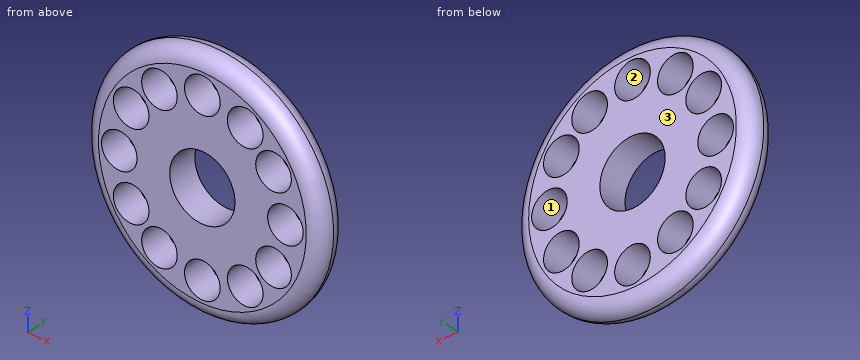
```python
from build123d import *

# Parameters (mm, degrees)
F0_R     = 40
F1_DEPTH = 5
F3_D     = 22
F4_D     = 12
F5_R     = 4.99999


# Not quite as in the source:
# - a fillet or chamfer is up to 0.001 mm smaller than in the source, because OpenCascade refuses the exact size
# - a feature names something its author has since deleted; it is built from what else it names


with BuildPart() as f1:
    # F0 (on Front) → F1 (new body, symmetric)
    with BuildSketch(Plane.XZ):
        Circle(F0_R)
    extrude(amount=F1_DEPTH, both=True)

    # F3 (through all)
    with Locations(Plane.XZ.offset(5)):
        with Locations((0, 0)):
            Hole(F3_D / 2)

    # F4 (through all)
    with Locations(Plane.XZ.offset(5)):
        with Locations((-28, 0), (0, 28), (28, 0), (0, -28), (-23.9821428571, 14.4518796002), (-14.4518796002, 23.9821428571), (14.4518796002, 23.9821428571), (23.9821428571, 14.4518796002), (23.9821428571, -14.4518796002), (-14.4518796002, -23.9821428571), (14.4518796002, -23.9821428571), (-23.9821428571, -14.4518796002)):
            Hole(F4_D / 2)

    # F5 (radius 5 in the source; OpenCascade refuses exactly that, so slightly less here)
    f5_edges = [f1.edges().sort_by_distance(p)[0] for p in [
        (-40, -5, 0),
        (-40, 5, 0),
        (40, 0, 0),
    ]]
    fillet(f5_edges, radius=F5_R)


solid = f1.part
```
Check sheet for the modelled part. Datum: model origin and axes. Units: mm. Face numbers are marked on the shaded views. Give positions to 0.01 mm unless a question says otherwise; leave off trailing zeros. Answer as a JSON object with one key per item and string values. Group by question number.
1) Depth check by flat-ended pin: P1, Ø15.5, axis at x = -23.98, z = 14.45, coming from the -Y side; P2, Ø5, axis at y = -3.5, z = 18.5, coming from the +X side; P3, Ø1, axis at y = -4, z = 7.5, coming from the -X side; P4, Ø7, axis at x = 14.45, z = -23.98, coming from the -Y side. Enter the tip coordinate at first touch or a pass-through.
2) Thickness scan on probe 1 along Z at (x, y) = (-19.5, 4); probe 2 along X at (y, z) = (2.25, -16.5); probe 3 along X at (y, z) = (-4, -15.5). Record the ranges inside material, lowest first. Write a range as from..to.
3) Release check for a two-part mould opening along Z. For the marked faces 1, 2 and 3 record: pulls with the +Z half, pulls with the -Z half, needs draft (parallel to the pull), parting line crosses it, or undercut.
4) Sectioned sample at A-A (x = 0). Give the number of separate pieces and of enclosed holes in the cut face, then the cut area to 3 significant figures.
Geometry results:
{
 "1": {"P1": "stops at y = -5", "P2": "stops at x = 35.99", "P3": "stops at x = -37.84", "P4": "passes through"},
 "2": {"probe 1": "z = -32.62..-27.23, -20.74..-18.44, -10.46..10.46, 18.44..20.74, 27.23..32.62", "probe 2": "x = -35.85..-29.62, -18.34..18.34, 29.62..35.85", "probe 3": "x = -34.7..-29.89, -18.07..18.07, 29.89..34.7"},
 "3": {"face 1": "undercut", "face 2": "undercut", "face 3": "needs draft"},
 "4": {"separate pieces": "4", "enclosed holes": "0", "area": "319 mm^2"}
}
